Input: part model. Units: mm. Frame: model coordinates. Coordinates: 2 decimals unless noted, no trailing zeros. Loops run counter-clockwise (first coordinate to the right, second up) from the corner with the lowest first, then second, coordinate; pieces in that order, holes last. Notation, with made-up numbers: (40, 38) -> (67, 38) arc R13 ccw to (67, 46) -> close; hole circle Ø6 at (37, 87.5). An arc over 180 degrees is marked (long way). Answer as a JSON object with one key per item and string values.
from build123d import *

# Parameters (mm, degrees)
SKETCH1_R           = 10
SKETCH1_R_2         = 7
BOSS_EXTRUDE1_DEPTH = 100
BOSS_EXTRUDE2_DEPTH = 100


with BuildPart() as part:
    # Sketch1 → Boss-Extrude1 (new body)
    with BuildSketch(Plane(origin=(0, 0, 0), x_dir=(1, 0, 0), z_dir=(0, 1, 0))):
        Circle(SKETCH1_R)
        Circle(SKETCH1_R_2, mode=Mode.SUBTRACT)
    extrude(amount=BOSS_EXTRUDE1_DEPTH)

    # Sketch2 → Boss-Extrude2 (add)
    with BuildSketch(Plane(origin=(0, 100, 0), x_dir=(1, 0, 0), z_dir=(0, 1, 0))):
        with BuildLine():
            Line((0, 10), (-5, 10))
            Line((-5, 10), (-5, 8.660254038))
            ThreePointArc((-5, 8.660254038), (-2.588190451, 9.659258263), (0, 10))
        make_face()
        with BuildLine():
            Line((5, 10), (0, 10))
            ThreePointArc((0, 10), (2.588190451, 9.659258263), (5, 8.660254038))
            Line((5, 8.660254038), (5, 10))
        make_face()
        with BuildLine():
            ThreePointArc((-1.3e-08, -10), (-2.588190457, -9.659258261), (-5, -8.660254038))
            Line((-5, -8.660254038), (-5, -10))
            Line((-5, -10), (-1.3e-08, -10))
        make_face()
        with BuildLine():
            Line((5, -10), (5, -8.660254038))
            ThreePointArc((5, -8.660254038), (2.588190445, -9.659258265), (-1.3e-08, -10))
            Line((-1.3e-08, -10), (5, -10))
        make_face()
    extrude(amount=-BOSS_EXTRUDE2_DEPTH)


solid = part.part
1. Section query A-A (x = 0). Return loops of the section in (y, z), plus the area to 3 significant figures.
Reply:
{"outline": "(0, -10) -> (100, -10) -> (100, -7) -> (0, -7) -> close; (0, 7) -> (100, 7) -> (100, 10) -> (0, 10) -> close", "area": "600 mm2"}
2. Pin query (flat end, axial travel): P1, Ø1.5, axis at y = 68.5, z = -9.5, coming from the -X side; P2, Ø5, axis at y = 74, z = -5.5, coming from the -X side; P3, Ø0.7, axis at y = 38, z = -9.5, coming from the +X side; P4, Ø1.5, axis at x = -1.5, z = 4.5, coming from the +Y side. Return the tip coordinate at first contact, or that it passes through.
Reply:
{"P1": "stops at x = -5", "P2": "stops at x = -9.54", "P3": "stops at x = 5", "P4": "passes through"}
3. Line query: line 1 along Z through (x, y) = (0, 53); line 2 along X through (y, z) = (48, -5); line 3 along X through (y, z) = (26.5, -6). Output: solid intervals per line, ascending.
Reply:
{"line 1": "z = -10 to -7, 7 to 10", "line 2": "x = -8.66 to -4.9, 4.9 to 8.66", "line 3": "x = -8 to -3.61, 3.61 to 8"}
4. Section query C-C (y = 70). Return loops of the section in (x, z).
Reply:
{"outline": "(-5, -10) -> (5, -10) -> (5, -8.66) arc R10 ccw to (5, 8.66) -> (5, 10) -> (-5, 10) -> (-5, 8.66) arc R10 ccw to (-5, -8.66) -> close; hole circle Ø14 at (0, 0)"}
5. Section query B-B (z = 0). Return loops of the section in (x, y).
Reply:
{"outline": "(-10, 0) -> (-7, 0) -> (-7, 100) -> (-10, 100) -> close; (7, 0) -> (10, 0) -> (10, 100) -> (7, 100) -> close"}
6. Section query D-D (x = 8.25). Return loops of the section in (y, z).
Reply:
{"outline": "(0, -5.65) -> (100, -5.65) -> (100, 5.65) -> (0, 5.65) -> close"}
7. Mould query, pull axis X, two halves, no side actions, for faces 1 (the face through (-10, 49, 0)), 2 (the face through (0, 51, -10)), 3 (the face through (6.466, 49.3, 2.681)). Classes: pulls with the +X half, pulls with the -X half, needs draft (parallel to the pull), parting line crosses it, or undercut.
Reply:
{"face 1": "pulls with the -X half", "face 2": "needs draft", "face 3": "undercut"}
